Could you check a few things on this model? Use its own coordinates, in mm. A direction names the side the tool comes from. Give positions to 0.01 mm unless a question says otherwise; leave off trailing zeros. Loops run counter-clockwise (first coordinate to the right, second up) from the corner with the lowest first, then second, coordinate; pieces in that order, holes last. Notation, with made-up numbers: (9.25, 50.25) -> (60.25, 50.25) arc R8 cw to (60.25, 54.25) -> close; hole circle Ø10 at (34, -31). An arc over 180 degrees is marked (long way). Write item = value, one per line. Start each with the question number.
1) I'm going to push flat-ended pins straight in: pin 1 Ø2 at (x, z) = (75.5, -36.5) entering from +Y; pin 2 Ø1 at (x, z) = (3, -26) entering from -Y; pin 3 Ø1 at (x, z) = (100, -7) entering from -Y. Where does each tip first touch, or does it pass through?
2) I want a section at C-C (y = -12.5). List the corners of the cut face in (x, z) for me, and give its area (3 significant figures).
3) I need wall thicknesses on probe 1 along Z at (x, y) = (142.5, -20.75); probe 2 along Z at (x, y) = (134, -15.4); probe 3 along X at (y, z) = (-18.25, -12). Which ranges of each line are inside material? Lowest first, please. Write a range as from..to.
4) If we mould it in two halves opening along X, with no side actions, what happens to faces 5 (the face through (82, -15, 0)), 6 (the face through (98.5, -25, -17)), 7 (the face through (163, -29, -43)), 8 (the face through (164.9, -14.8, -44))? For each: +X half, -X half, draft (parallel to the pull), parting line (faces both ways), or undercut.
5) I want a section at B-B (x = 61). List the corners of the cut face in (y, z) for me, and give its area (3 significant figures).
6) On a 3-axis mill with a long thin cutter (end or side, diameter ignored), from which of +Z, -Z, +X, -X, +Y, -Y can I reach the whole of each face in a straight line? I mean faces 1 (the face through (161, -10.5, -6.1)), 2 (the face through (105, -23, -10)), 3 (the face through (144, -3, -23)), 4 (the face through (98, -22, -19)). Say none if no direction works.
7) I want a section at D-D (y = -5.25). List the corners of the cut face in (x, z) for me, and give its area (3 significant figures).
8) I want a section at A-A (z = -23). List the corners of the cut face in (x, y) for me.
from build123d import *

# Parameters (mm, degrees)
SKETCH_R        = 8
SKETCH_W        = 130
SKETCH_H        = 32
PAD_DEPTH       = 7
PAD001_DEPTH    = 7
SKETCH003_W     = 26
SKETCH003_H     = 24
SKETCH003_R     = 3.5
PAD002_DEPTH    = 3
SKETCH004_R     = 1.5
SKETCH004_W     = 159
SKETCH004_H     = 14
PAD003_DEPTH    = 4
PAD004_DEPTH    = 10
POCKET_DEPTH    = 7
POCKET001_DEPTH = 10
PAD005_DEPTH    = 2
SKETCH009_R     = 1
POCKET002_DEPTH = 10


with BuildPart() as part:
    # Sketch → Pad (new body)
    with BuildSketch(Plane.XZ):
        with BuildLine():
            ThreePointArc((7, 0), (2.050253, -2.050253), (0, -7))
            Line((0, -39), (0, -7))
            ThreePointArc((0, -39), (2.050253, -43.949747), (7, -46))
            Line((160, -46), (7, -46))
            ThreePointArc((160, -46), (164.949747, -43.949747), (167, -39))
            Line((167, -7), (167, -39))
            ThreePointArc((167, -7), (164.949747, -2.050253), (160, 0))
            Line((7, 0), (160, 0))
        make_face()
        with Locations((152, -23)):
            Circle(SKETCH_R, mode=Mode.SUBTRACT)
        with Locations((72, -23)):
            Rectangle(SKETCH_W, SKETCH_H, mode=Mode.SUBTRACT)
    extrude(amount=PAD_DEPTH)

    # Sketch002 (on Face15 of Pad) → Pad001 (join)
    with BuildSketch(Plane.XZ.offset(7)):
        with BuildLine():
            ThreePointArc((7, 0), (2.050253, -2.050253), (0, -7))
            Line((0, -39), (0, -7))
            ThreePointArc((0, -39), (2.050253, -43.949747), (7, -46))
            Line((160, -46), (7, -46))
            ThreePointArc((160, -46), (164.949747, -43.949747), (167, -39))
            Line((167, -7), (167, -39))
            ThreePointArc((167, -7), (164.949747, -2.050253), (160, 0))
            Line((7, 0), (160, 0))
        make_face()
        with BuildLine():
            ThreePointArc((11, -4), (6.050253, -6.050253), (4, -11))
            Line((4, -35), (4, -11))
            ThreePointArc((4, -35), (6.050253, -39.949747), (11, -42))
            Line((156, -42), (11, -42))
            ThreePointArc((156, -42), (160.949747, -39.949747), (163, -35))
            Line((163, -11), (163, -35))
            ThreePointArc((163, -11), (160.949747, -6.050253), (156, -4))
            Line((11, -4), (156, -4))
        make_face(mode=Mode.SUBTRACT)
    extrude(amount=PAD001_DEPTH)

    # Sketch003 (on Face24 of Pad001) → Pad002 (join)
    with BuildSketch(Plane.XZ.offset(7)):
        with Locations((150, -23)):
            Rectangle(SKETCH003_W, SKETCH003_H)
        with Locations((152, -23)):
            Circle(SKETCH003_R, mode=Mode.SUBTRACT)
    extrude(amount=PAD002_DEPTH)

    # Sketch004 (on Face18 of Pad002) → Pad003 (join)
    with BuildSketch(Plane.XZ.offset(14)):
        with BuildLine():
            ThreePointArc((7, 0), (2.050253, -2.050253), (0, -7))
            Line((0, -39), (0, -7))
            ThreePointArc((0, -39), (2.050253, -43.949747), (7, -46))
            Line((160, -46), (7, -46))
            ThreePointArc((160, -46), (164.949747, -43.949747), (167, -39))
            Line((167, -7), (167, -39))
            ThreePointArc((167, -7), (164.949747, -2.050253), (160, 0))
            Line((7, 0), (160, 0))
        make_face()
        with Locations((10, -13)):
            Circle(SKETCH004_R, mode=Mode.SUBTRACT)
        with Locations((10, -33)):
            Circle(SKETCH004_R, mode=Mode.SUBTRACT)
        with Locations((134, -13)):
            Circle(SKETCH004_R, mode=Mode.SUBTRACT)
        with Locations((134, -33)):
            Circle(SKETCH004_R, mode=Mode.SUBTRACT)
        with Locations((83.5, -23)):
            Rectangle(SKETCH004_W, SKETCH004_H, mode=Mode.SUBTRACT)
    extrude(amount=PAD003_DEPTH)

    # Sketch005 (on Face29 of Pad003) → Pad004 (join)
    with BuildSketch(Plane.XZ.offset(18)):
        with BuildLine():
            ThreePointArc((7, 0), (2.050253, -2.050253), (0, -7))
            Line((0, -39), (0, -7))
            ThreePointArc((0, -39), (2.050253, -43.949747), (7, -46))
            Line((160, -46), (7, -46))
            ThreePointArc((160, -46), (164.949747, -43.949747), (167, -39))
            Line((167, -7), (167, -39))
            ThreePointArc((167, -7), (164.949747, -2.050253), (160, 0))
            Line((7, 0), (160, 0))
        make_face()
        with BuildLine():
            ThreePointArc((11, -4), (6.050253, -6.050253), (4, -11))
            Line((4, -35), (4, -11))
            ThreePointArc((4, -35), (6.050253, -39.949747), (11, -42))
            Line((11, -42), (15, -42))
            Line((15, -42), (15, -27))
            Line((15, -27), (35, -27))
            Line((35, -27), (35, -43))
            Line((35, -43), (95, -43))
            Line((95, -27), (95, -43))
            Line((95, -27), (105, -27))
            Line((105, -27), (105, -42))
            Line((105, -42), (140, -42))
            Line((140, -42), (140, -27))
            Line((140, -27), (145, -27))
            Line((145, -27), (145, -42))
            Line((145, -42), (156, -42))
            ThreePointArc((156, -42), (160.949747, -39.949747), (163, -35))
            Line((163, -11), (163, -35))
            ThreePointArc((163, -11), (160.949747, -6.050253), (156, -4))
            Line((145, -4), (156, -4))
            Line((145, -19), (145, -4))
            Line((140, -19), (145, -19))
            Line((140, -4), (140, -19))
            Line((105, -4), (140, -4))
            Line((105, -19), (105, -4))
            Line((95, -19), (105, -19))
            Line((95, -3), (95, -19))
            Line((35, -3), (95, -3))
            Line((35, -3), (35, -19))
            Line((15, -19), (35, -19))
            Line((15, -4), (15, -19))
            Line((11, -4), (15, -4))
        make_face(mode=Mode.SUBTRACT)
    extrude(amount=PAD004_DEPTH)

    # Sketch006 (on Face48 of Pad004) → Pocket (cut)
    with BuildSketch(Plane.XZ.offset(28)):
        Polygon((2, -14), (30, -14), (30, -23), (30, -32), (2, -32), align=None)
        Polygon((98.5, -14), (142.5, -14), (142.5, -23), (142.5, -32), (98.5, -32), align=None)
    extrude(amount=-POCKET_DEPTH, mode=Mode.SUBTRACT)

    # Sketch007 (on Face33 of Pocket) → Pocket001 (cut)
    with BuildSketch(Plane(origin=(0, 0, 0), x_dir=(0, 0, -1), z_dir=(-1, 0, 0))):
        with BuildLine():
            ThreePointArc((19.25, 26.5), (18.542893, 26.207107), (18.25, 25.5))
            Line((18.25, 24.75), (18.25, 25.5))
            Line((18.25, 24), (18.25, 24.75))
            ThreePointArc((18.25, 24), (18.542893, 23.292893), (19.25, 23))
            Line((26.75, 23), (19.25, 23))
            ThreePointArc((26.75, 23), (27.457107, 23.292893), (27.75, 24))
            Line((27.75, 25.5), (27.75, 24))
            ThreePointArc((27.75, 25.5), (27.457107, 26.207107), (26.75, 26.5))
            Line((23, 26.5), (26.75, 26.5))
            Line((19.25, 26.5), (23, 26.5))
        make_face()
    extrude(amount=-POCKET001_DEPTH, mode=Mode.SUBTRACT)

    # Sketch008 (on Face48 of Pocket001) → Pad005 (join)
    with BuildSketch(Plane.XZ.offset(28)):
        with BuildLine():
            ThreePointArc((7, 0), (2.050253, -2.050253), (0, -7))
            Line((0, -39), (0, -7))
            ThreePointArc((0, -39), (2.050253, -43.949747), (7, -46))
            Line((160, -46), (7, -46))
            ThreePointArc((160, -46), (164.949747, -43.949747), (167, -39))
            Line((167, -7), (167, -39))
            ThreePointArc((167, -7), (164.949747, -2.050253), (160, 0))
            Line((7, 0), (160, 0))
        make_face()
        with BuildLine():
            ThreePointArc((7, -2), (3.464466, -3.464466), (2, -7))
            Line((2, -39), (2, -7))
            ThreePointArc((2, -39), (3.464466, -42.535534), (7, -44))
            Line((160, -44), (7, -44))
            ThreePointArc((160, -44), (163.535534, -42.535534), (165, -39))
            Line((165, -7), (165, -39))
            ThreePointArc((165, -7), (163.535534, -3.464466), (160, -2))
            Line((7, -2), (160, -2))
        make_face(mode=Mode.SUBTRACT)
    extrude(amount=PAD005_DEPTH)

    # Sketch009 (on Face111 of Pad005) → Pocket002 (cut)
    with BuildSketch(Plane.XZ.offset(28)):
        with Locations((25, -7)):
            Circle(SKETCH009_R)
        with Locations((100, -7)):
            Circle(SKETCH009_R)
        with Locations((142.5, -7)):
            Circle(SKETCH009_R)
        with Locations((25, -39)):
            Circle(SKETCH009_R)
        with Locations((100, -39)):
            Circle(SKETCH009_R)
        with Locations((142.5, -39)):
            Circle(SKETCH009_R)
    extrude(amount=-POCKET002_DEPTH, mode=Mode.SUBTRACT)


solid = part.part
Answer list:
q1.pin_1 = -14
q1.pin_2 = -21
q1.pin_3 = -18
q2.outline = (0, -39) arc R7 ccw to (7, -46) -> (160, -46) arc R7 ccw to (167, -39) -> (167, -7) arc R7 ccw to (160, 0) -> (7, 0) arc R7 ccw to (0, -7) -> close; hole (4, -35) arc R7 ccw to (11, -42) -> (156, -42) arc R7 ccw to (163, -35) -> (163, -11) arc R7 ccw to (156, -4) -> (11, -4) arc R7 ccw to (4, -11) -> close
q2.area = 1,640 mm^2
q3.probe_1 = -46..-40, -38..-27, -19..-8, -6..0
q3.probe_2 = -46..-34.5, -31.5..-30, -16..-14.5, -11.5..0
q3.probe_3 = 0..4, 15..35, 95..105, 140..145, 163..167
q4.face_5 = draft
q4.face_6 = undercut
q4.face_7 = undercut
q4.face_8 = +X half
q5.outline = (-30, -46) -> (0, -46) -> (0, -39) -> (-7, -39) -> (-7, -42) -> (-14, -42) -> (-14, -30) -> (-18, -30) -> (-18, -43) -> (-28, -43) -> (-28, -44) -> (-30, -44) -> close; (-30, -2) -> (-28, -2) -> (-28, -3) -> (-18, -3) -> (-18, -16) -> (-14, -16) -> (-14, -4) -> (-7, -4) -> (-7, -7) -> (0, -7) -> (0, 0) -> (-30, 0) -> close
q5.area = 350 mm^2
q6.face_1 = none
q6.face_2 = -Y
q6.face_3 = +Y
q6.face_4 = +Y, -Y
q7.outline = (0, -39) arc R7 ccw to (7, -46) -> (160, -46) arc R7 ccw to (167, -39) -> (167, -7) arc R7 ccw to (160, 0) -> (7, 0) arc R7 ccw to (0, -7) -> close; hole (7, -39) -> (137, -39) -> (137, -7) -> (7, -7) -> close; hole circle Ø16 at (152, -23)
q7.area = 3,280 mm^2
q8.outline = (0, -30) -> (2, -30) -> (2, -26.5) -> (0, -26.5) -> close; (0, -23) -> (2, -23) -> (2, -21) -> (4, -21) -> (4, -7) -> (7, -7) -> (7, 0) -> (0, 0) -> close; (137, -10) -> (148.5, -10) -> (148.5, -7) -> (144, -7) -> (144, 0) -> (137, 0) -> close; (155.5, -10) -> (163, -10) -> (163, -28) -> (165, -28) -> (165, -30) -> (167, -30) -> (167, 0) -> (160, 0) -> (160, -7) -> (155.5, -7) -> close
